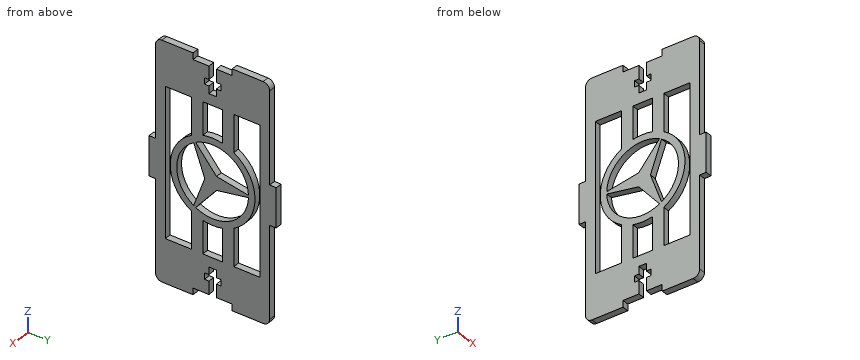
from build123d import *

# Parameters (mm, degrees)
BOSS_EXTRUDE1_DEPTH = 2.54
FILLET1_R           = 2.54
CUT_EXTRUDE2_REACH  = 4.54
CUT_EXTRUDE3_DEPTH  = 2.54


with BuildPart() as part:
    # Sketch2 → Boss-Extrude1 (new body)
    with BuildSketch(Plane(origin=(0, 0, 0), x_dir=(0, 0, -1), z_dir=(1, 0, 0))):
        Polygon((-45.72, 22.225), (-45.72, 7.62), (-43.18, 7.62), (-43.18, 1.4478), (-38.1, 1.4478), (-38.1, 3.175), (-35.66795, 3.175), (-35.66795, 1.4478), (-32.766, 1.4478), (-32.766, -1.4478), (-35.66795, -1.4478), (-35.66795, -3.175), (-38.1, -3.175), (-38.1, -1.4478), (-43.18, -1.4478), (-43.18, -7.62), (-45.72, -7.62), (-45.72, -22.225), (-7.62, -22.225), (-7.62, -24.765), (7.62, -24.765), (7.62, -22.225), (45.72, -22.225), (45.72, -7.62), (43.18, -7.62), (43.18, -1.4478), (38.1, -1.4478), (38.1, -3.175), (35.66795, -3.175), (35.66795, -1.4478), (32.766, -1.4478), (32.766, 1.4478), (35.66795, 1.4478), (35.66795, 3.175), (38.1, 3.175), (38.1, 1.4478), (43.18, 1.4478), (43.18, 7.62), (45.72, 7.62), (45.72, 22.225), (7.62, 22.225), (7.62, 24.765), (-7.62, 24.765), (-7.62, 22.225), align=None)
    extrude(amount=BOSS_EXTRUDE1_DEPTH)

    # Fillet1
    fillet1_edges = [part.edges().sort_by_distance(p)[0] for p in [
        (1.27, -22.225, -45.72),
        (1.27, -22.225, 45.72),
        (1.27, 22.225, 45.72),
        (1.27, 22.225, -45.72),
    ]]
    fillet(fillet1_edges, radius=FILLET1_R)

    # Sketch3 → Cut-Extrude2 (cut, up to next)
    with BuildSketch(Plane(origin=(2.54, 0, 0), x_dir=(0, 0, -1), z_dir=(1, 0, 0)), mode=Mode.PRIVATE) as cut_extrude2_sk1:
        with BuildLine():
            Line((2.639645431, 1.524), (12.316467203, -6.592839725))
            ThreePointArc((12.316467203, -6.592839725), (12.098374891, 6.985), (0.448666916, 13.962793345))
            Line((0.448666916, 13.962793345), (2.639645431, 1.524))
        make_face()
    cut_extrude2_tool1 = extrude(cut_extrude2_sk1.sketch, amount=-CUT_EXTRUDE2_REACH, mode=Mode.PRIVATE) & part.part
    add(cut_extrude2_tool1.solids().sort_by_distance((2.54, 4.379888, -7.586189))[0], mode=Mode.SUBTRACT)
    # Sketch3 → Cut-Extrude2 (cut, up to next)
    with BuildSketch(Plane(origin=(2.54, 0, 0), x_dir=(0, 0, -1), z_dir=(1, 0, 0)), mode=Mode.PRIVATE) as cut_extrude2_sk2:
        with BuildLine():
            Line((0, -3.048), (11.867800287, -7.36995362))
            ThreePointArc((11.867800287, -7.36995362), (0, -13.97), (-11.867800287, -7.36995362))
            Line((-11.867800287, -7.36995362), (0, -3.048))
        make_face()
    cut_extrude2_tool2 = extrude(cut_extrude2_sk2.sketch, amount=-CUT_EXTRUDE2_REACH, mode=Mode.PRIVATE) & part.part
    add(cut_extrude2_tool2.solids().sort_by_distance((2.54, -8.759776, 0))[0], mode=Mode.SUBTRACT)
    # Sketch3 → Cut-Extrude2 (cut, up to next)
    with BuildSketch(Plane(origin=(2.54, 0, 0), x_dir=(0, 0, -1), z_dir=(1, 0, 0)), mode=Mode.PRIVATE) as cut_extrude2_sk3:
        with BuildLine():
            Line((-2.639645431, 1.524), (-0.448666916, 13.962793345))
            ThreePointArc((-0.448666916, 13.962793345), (-12.098374891, 6.985), (-12.316467203, -6.592839725))
            Line((-12.316467203, -6.592839725), (-2.639645431, 1.524))
        make_face()
    cut_extrude2_tool3 = extrude(cut_extrude2_sk3.sketch, amount=-CUT_EXTRUDE2_REACH, mode=Mode.PRIVATE) & part.part
    add(cut_extrude2_tool3.solids().sort_by_distance((2.54, 4.379888, 7.586189))[0], mode=Mode.SUBTRACT)

    # Sketch4 → Cut-Extrude3 (cut)
    with BuildSketch(Plane(origin=(2.54, 0, 0), x_dir=(0, 0, -1), z_dir=(1, 0, 0))):
        with BuildLine():
            Line((-28.764370514, 18.415), (28.764370514, 18.415))
            Line((28.764370514, 18.415), (28.764370514, 8.255))
            Line((28.764370514, 8.255), (14.298079416, 8.255))
            ThreePointArc((14.298079416, 8.255), (0, 16.51), (-14.298079416, 8.255))
            Line((-14.298079416, 8.255), (-28.764370514, 8.255))
            Line((-28.764370514, 8.255), (-28.764370514, 18.415))
        make_face()
        with BuildLine():
            Line((-28.764370514, -18.415), (-28.764370514, -8.255))
            Line((-28.764370514, -8.255), (-14.298079416, -8.255))
            ThreePointArc((-14.298079416, -8.255), (0, -16.51), (14.298079416, -8.255))
            Line((14.298079416, -8.255), (28.764370514, -8.255))
            Line((28.764370514, -8.255), (28.764370514, -18.415))
            Line((28.764370514, -18.415), (-28.764370514, -18.415))
        make_face()
        with BuildLine():
            Line((-16.064370514, 3.81), (-28.764370514, 3.81))
            Line((-28.764370514, 3.81), (-28.764370514, -3.81))
            Line((-28.764370514, -3.81), (-16.064370514, -3.81))
            ThreePointArc((-16.064370514, -3.81), (-16.51, 0), (-16.064370514, 3.81))
        make_face()
        with BuildLine():
            Line((28.764370514, -3.81), (16.064370514, -3.81))
            ThreePointArc((16.064370514, -3.81), (16.51, 0), (16.064370514, 3.81))
            Line((16.064370514, 3.81), (28.764370514, 3.81))
            Line((28.764370514, 3.81), (28.764370514, -3.81))
        make_face()
    extrude(amount=-CUT_EXTRUDE3_DEPTH, mode=Mode.SUBTRACT)


solid = part.part
Build history of the part. All positions in model axes, mm. Give positions to 0.01 mm unless a question says otherwise; leave off trailing zeros. Write each loop counter-clockwise with the first axis right and the second up, starting at its lowest first coordinate (ties: lowest second). Pieces come first, ordered by that corner, then holes. Notation, with made-up numbers: (-6.75, 69) - (26.25, 69) arc R29 cw to (26.25, 101) - close; hole circle Ø4 at (-22.5, -13). An arc over 180 degrees is marked (long way). Use one line per item in the form item = value. Start each with the question number.
1. Drop flat-ended pins along their axis: pin 1 Ø0.8 at (x, z) = (1, -24) entering from +Y (3 decimals); pin 2 Ø1.2 at (x, z) = (1, -37) entering from -Y (3 decimals); pin 3 Ø0.5 at (x, y) = (1.5, -2) entering from +Z; pin 4 Ø3 at (y, z) = (-2, 12) entering from +X. Give the stop position or say it passes through.
2. Probe line 1 (Y direction, x = 1.8, z = 17) (3 decimals); line 2 (Y direction, x = 1.3, z = 38) (3 decimals); line 3 (Z direction, x = 0.4, y = 17.5). List the from-to ranges inside material, lowest first. Write a range as [from, to].
3. Band-saw the part on C-C on z = -31. Write the cut outline in (x, y) (3 decimals).
4. Band-saw the part on B-B on x = 2.05. Count the separate pieces of the cut face and the enclosed holes in it, plus the area to 3 significant figures.
5. Band-saw the part on A-A on z = 22. Write the cut outline in (x, y) (3 decimals).
Conclusion:
q1.pin_1 = 22.225
q1.pin_2 = -22.225
q1.pin_3 = 43.18
q1.pin_4 = through
q2.line_1 = [-22.225, -18.415], [-8.255, -3.81], [3.81, 8.255], [18.415, 22.225]
q2.line_2 = [-22.225, -3.175], [3.175, 22.225]
q2.line_3 = [-45.72, -28.76], [28.76, 45.72]
q3.outline = (0, -22.225) - (2.54, -22.225) - (2.54, 22.225) - (0, 22.225) - close
q4.separate_pieces = 1
q4.enclosed_holes = 7
q4.area = 2,470 mm²
q5.outline = (0, -22.225) - (2.54, -22.225) - (2.54, -18.415) - (0, -18.415) - close; (0, -8.255) - (2.54, -8.255) - (2.54, -3.81) - (0, -3.81) - close; (0, 3.81) - (2.54, 3.81) - (2.54, 8.255) - (0, 8.255) - close; (0, 18.415) - (2.54, 18.415) - (2.54, 22.225) - (0, 22.225) - close
